Geometry: see drawing. Coordinates: mm, zero at the bounding-box minimum. A direction names the side the tool comes from. Give positions to 0.01 mm unless a question says otherwise; leave off trailing zeros. Loops run counter-clockwise (first coordinate to the right, second up) from the corner with the lowest first, then second, coordinate; pieces in that order, holes last. Notation, with made-up numbers: M 70,22 L 98,22 A22 ccw 98,57 Z; hole C 2.5,85.5 d3. An arc over 180 degrees is marked long. Answer in a Markdown table with one row per item.
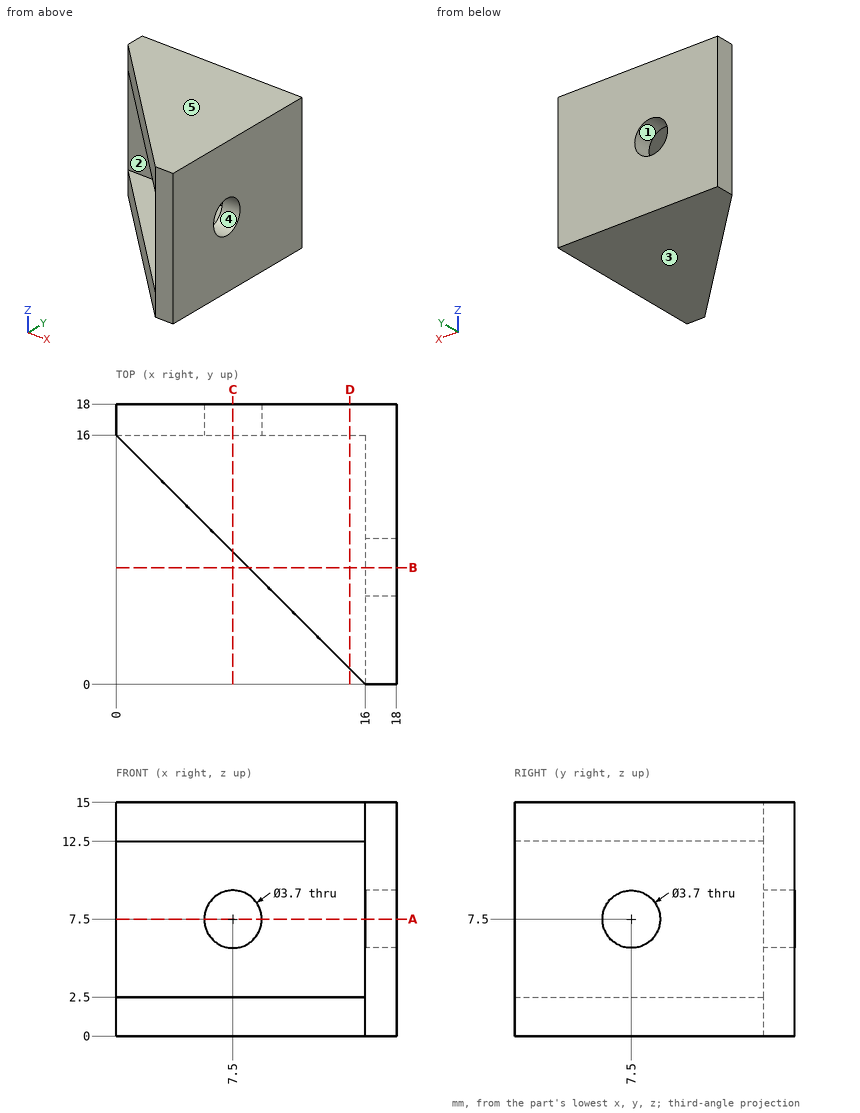
1) Section A-A, the plane z = 7.5. Return loops of the section in (x, y), then the cut area to 3 significant figures.
Reply:
| item | result |
|---|---|
| outline | M 0,16 L 5.65,16 L 5.65,18 L 0,18 Z; M 9.35,16 L 16,16 L 16,9.35 L 18,9.35 L 18,18 L 9.35,18 Z; M 16,0 L 18,0 L 18,5.65 L 16,5.65 Z |
| area | 53.2 mm² |
2) Section D-D, the plane x = 15. Return loops of the section in (y, z).
Reply:
| item | result |
|---|---|
| outline | M 1,0 L 18,0 L 18,15 L 1,15 L 1,12.5 L 16,12.5 L 16,2.5 L 1,2.5 Z |
3) Pull-direction query (Z, two-part tool) for the marked faces 3, 4 and 5; classes: released by +Z, released by -Z, zero draft, split by the parting line, or undercut.
Reply:
| item | result |
|---|---|
| face 3 | released by -Z |
| face 4 | undercut |
| face 5 | released by +Z |
4) Material intervals for L1, parallel to Z at x = 13, y = 10.5; L2, parallel to Y at x = 16.6, z = 7.5, sorted ascending.
Reply:
| item | result |
|---|---|
| L1 | z = 0 to 2.5, 12.5 to 15 |
| L2 | y = 0 to 5.65, 9.35 to 18 |
5) Section B-B, the plane y = 7.5. Return loops of the section in (x, z).
Reply:
| item | result |
|---|---|
| outline | M 8.5,0 L 18,0 L 18,5.65 L 16,5.65 L 16,2.5 L 8.5,2.5 Z; M 8.5,12.5 L 16,12.5 L 16,9.35 L 18,9.35 L 18,15 L 8.5,15 Z |
6) Pin query (flat end, axial travel): pin 1 Ø1.5 at (y, z) = (9.5, 11.5) entering from -X; pin 2 Ø6 at (y, z) = (7, 13.5) entering from -X; pin 3 Ø8 at (y, z) = (5, 9.5) entering from -X; pin 4 Ø3.5 at (x, z) = (7.5, 7.5) entering from +Y. Return the tip coordinate at first contact, or that it passes through.
Reply:
| item | result |
|---|---|
| pin 1 | stops at x = 16 |
| pin 2 | stops at x = 6 |
| pin 3 | stops at x = 8.35 |
| pin 4 | passes through |
7) Set-up query: the marked faces 1 and 2. Return all of +Z, -Z, +X, -X, +Y, -Y with unobstructed straight access to the full face (end or side cutting, diameter ignored); none if empty.
Reply:
| item | result |
|---|---|
| face 1 | +Y, -Y |
| face 2 | -X, -Y |
